from build123d import *

# Parameters (mm, degrees)
F0_R     = 31.75
F0_R_2   = 17.4625
F1_DEPTH = 25.4
F0_R_3   = 15.875
F2_DEPTH = 50.8
F3_SIZE  = 13.97
F6_DEPTH = 9.525
F10_D    = 3.175
F13_D    = 3.175


# Not quite as in the source:
# - a fillet or chamfer that OpenCascade refuses, or shapes differently, is made with other operations: its cross-section is extruded or revolved along the edge and cut away or added


with BuildPart() as f1:
    # F0 (on Top) → F1 (new body)
    with BuildSketch(Plane.XY):
        Circle(F0_R)
        Circle(F0_R_2, mode=Mode.SUBTRACT)
    extrude(amount=-F1_DEPTH)

    # F0 (on Top) → F2 (join)
    with BuildSketch(Plane.XY):
        Circle(F0_R_2)
        Circle(F0_R_3, mode=Mode.SUBTRACT)
    extrude(amount=-F2_DEPTH)

    # F3
    f3_edges = [f1.edges().sort_by_distance(p)[0] for p in [
        (-31.75, 0, -25.4),
    ]]
    chamfer(f3_edges, length=F3_SIZE)

    # F4: fillet of radius 5.08 on 1 edges, made by hand

    # F4_s1 → F4_t2 (revolve, cut)
    with BuildSketch(Plane.XZ):
        with BuildLine():
            ThreePointArc((18.677323371, -24.502676629), (18.1034449464, -24.9967366519), (17.4625, -25.4))
            Line((17.4625, -25.4), (17.78, -25.4))
            Line((17.78, -25.4), (18.677323371, -24.502676629))
        make_face()
    revolve(axis=Axis((0, 0, -25.4), (0, 0, 1)), mode=Mode.SUBTRACT)

    # F5 (on Top) → F6 (cut)
    with BuildSketch(Plane.XY):
        with BuildLine():
            ThreePointArc((-5.715, 29.6161304233), (-21.3281082875, 21.3281082875), (-29.6161304233, 5.715))
            Line((-29.6161304233, 5.715), (-16.5008388044, 5.715))
            ThreePointArc((-16.5008388044, 5.715), (-12.3478521665, 12.3478521665), (-5.715, 16.5008388044))
            Line((-5.715, 16.5008388044), (-5.715, 29.6161304233))
        make_face()
        with BuildLine():
            ThreePointArc((-29.6161304233, -5.715), (-21.3281082875, -21.3281082875), (-5.715, -29.6161304233))
            Line((-5.715, -29.6161304233), (-5.715, -16.5008388044))
            ThreePointArc((-5.715, -16.5008388044), (-12.3478521665, -12.3478521665), (-16.5008388044, -5.715))
            Line((-16.5008388044, -5.715), (-29.6161304233, -5.715))
        make_face()
        with BuildLine():
            Line((5.715, -16.5008388044), (5.715, -29.6161304233))
            ThreePointArc((5.715, -29.6161304233), (21.3281082875, -21.3281082875), (29.6161304233, -5.715))
            Line((29.6161304233, -5.715), (16.5008388044, -5.715))
            ThreePointArc((16.5008388044, -5.715), (12.3478521665, -12.3478521665), (5.715, -16.5008388044))
        make_face()
        with BuildLine():
            Line((16.5008388044, 5.715), (29.6161304233, 5.715))
            ThreePointArc((29.6161304233, 5.715), (21.3281082875, 21.3281082875), (5.715, 29.6161304233))
            Line((5.715, 29.6161304233), (5.715, 16.5008388044))
            ThreePointArc((5.715, 16.5008388044), (12.3478521665, 12.3478521665), (16.5008388044, 5.715))
        make_face()
    extrude(amount=-F6_DEPTH, mode=Mode.SUBTRACT)

    # F10 (through all)
    with Locations(Plane.XZ.offset(50.8)):
        with Locations((0, -5.4679759778)):
            Hole(F10_D / 2)

    # F13 (through all)
    with Locations(Plane.YZ.offset(50.8)):
        with Locations((0, -5.3200940602)):
            Hole(F13_D / 2)


solid = f1.part
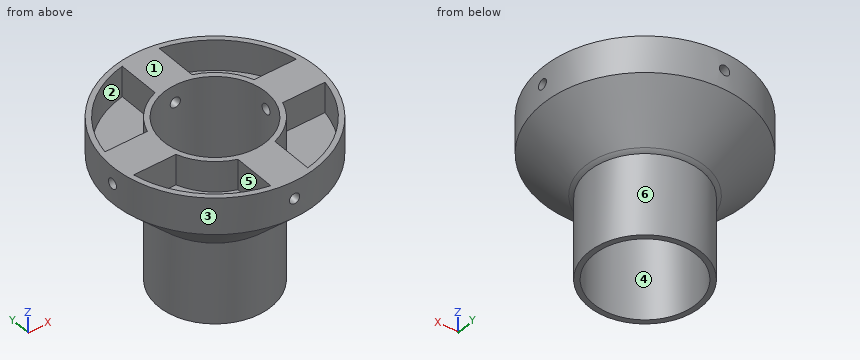
Could you check a few things on this model? Use its own coordinates, in mm. Face numbers are marked on the shaded views. A direction names the side the tool comes from. Coordinates: 2 decimals unless noted, no trailing zeros. Write each loop counter-clockwise with the first axis right and the second up, starting at its lowest first coordinate (ties: lowest second). Pieces come first, ordered by that corner, then holes. Notation, with made-up numbers: (72.25, 53.5) - (91.25, 53.5) arc R20 ccw to (91.25, 59.5) - close; hole circle Ø2 at (62.5, 61.25). An arc over 180 degrees is marked (long way). Put each result on its own line as item: value. Start each with the question number.
Q1. Thinking about a two-plate mould opening in X: for the marked faces 1, 2 and 3, which applies, pulls with the +X half, pulls with the -X half, needs draft (parallel to the pull), parting line crosses it, or undercut?
Q2. I want a section at A-A on x = 0. Count the separate pieces of the cut face and the enclosed holes in it, plus the area to 3 significant figures.
Q3. I'm going to push flat-ended pins straight in: P1, Ø3, axis at x = -21, y = -24.5, coming from the -Z side; P2, Ø1.5, axis at y = -10, z = -43, coming from the -X side; P3, Ø5, axis at x = 22.5, z = -6, coming from the -Y side. Where does each tip first touch, or does it pass through?
Q4. Which directions (+Z, -Z, +X, -X, +Y, -Y) give clear straight access to the entire face, cutting with the end or side of a thin tool? Please do the marked faces 4, 5 and 6.
Q5. I want a section at D-D on z = -13.5. Write out the boundary of the cut face in (x, y) (3 decimals), plus the area to 3 significant figures.
Q6. Please list where these lines run through material, in increasing order: L1, parallel to Y at x = -24, z = -4 (3 decimals); L2, parallel to Y at x = -26.5, z = -9 (1 decimal); L3, parallel to X at y = -23, z = -5 (1 decimal).
Checks:
1. face 1: needs draft
1. face 2: undercut
1. face 3: parting line crosses it
2. separate pieces: 4
2. enclosed holes: 0
2. area: 591 mm²
3. P1: z = -12.41
3. P2: x = -14.81
3. P3: y = -24.66
4. face 4: +Z, -Z
4. face 5: +Z
4. face 6: -Z
5. outline: circle Ø59.36 at (0, 0); hole circle Ø31.75 at (0, 0)
5. area: 1,980 mm²
6. L1: -20.786 to -18.27, -5.715 to -0.882, 0.882 to 5.715, 18.27 to 20.786
6. L2: -17.5 to -14.4, -5.7 to 5.7, 14.4 to 17.5
6. L3: -21.9 to -19.5, -5.7 to -1.5, 1.5 to 5.7, 19.5 to 21.9
